Could you check a few things on this model? Use its own coordinates, in mm. A direction names the side the tool comes from. Give positions to 0.01 mm unless a question says otherwise; leave off trailing zeros. Loops run counter-clockwise (first coordinate to the right, second up) from the corner with the lowest first, then second, coordinate; pieces in that order, holes last. Notation, with made-up numbers: (12, 40) - (59, 40) arc R38 cw to (59, 78) - close; hole circle Ø11 at (20, 2.25). An arc over 180 degrees is marked (long way). Write each question's results on one line, items separated by ' | '. Start each with the question number.
1) If I drill on probe 1 along Z at (x, y) = (-30.5, 0.5); probe 2 along X at (y, z) = (-2.5, 0.7) (3 decimals); probe 3 along X at (y, z) = (-4.25, 2.55), over which ranges is the centre line in solid material (lowest first)? Write a range as [from, to].
2) If we mould it in two halves opening along X, with no side actions, what happens to faces 1 (the face through (-47, 0, 1)), 2 (the face through (-1.7, -3.2, 1)), 3 (the face through (-38, -5, 2))? For each: +X half, -X half, draft (parallel to the pull), parting line (faces both ways), or undercut.
3) I want a section at B-B, the plane y = 0.5. Write out the boundary of the cut face in (x, z), and give its area (3 significant figures).
4) I want a section at C-C, the plane y = -1.5. Write out the boundary of the cut face in (x, z).
5) I want a section at A-A, the plane z = 1.35. Count the separate pieces of the cut face and the enclosed holes in it, and give its area (3 significant figures).
6) I want a section at D-D, the plane y = 2.5. Write out the boundary of the cut face in (x, z) (3 decimals), and give its area (3 significant figures).
7) On a 3-axis mill with a long thin cutter (end or side, diameter ignored), from which of +Z, -Z, +X, -X, +Y, -Y can I reach the whole of each face in a straight line? I mean faces 4 (the face through (-3, -5, 1)), 5 (the face through (-42, -4, 3)), 6 (the face through (-35, -4, 3)). Say none if no direction works.
8) I'm going to push a flat-ended pin straight in: pin 1 (2.5 mm diameter, centred on x = -9.625, y = 0, fed in from +Z). Where does the tip first touch, or does it pass through?
from build123d import *

# Parameters (mm, degrees)
BOSS_EXTRUDE1_DEPTH = 2
SKETCH3_R           = 3.625
SKETCH3_R_2         = 1
CUT_EXTRUDE1_DEPTH  = 2
SKETCH4_W           = 7
SKETCH4_H           = 4
BOSS_EXTRUDE2_DEPTH = 3
SKETCH7_R           = 2
CUT_EXTRUDE2_DEPTH  = 7


with BuildPart() as part:
    # Sketch1 → Boss-Extrude1 (new body)
    with BuildSketch(Plane.XY):
        with BuildLine():
            Line((-42, 5), (0, 5))
            ThreePointArc((0, 5), (5, 0), (0, -5))
            Line((0, -5), (-42, -5))
            ThreePointArc((-42, -5), (-47, 0), (-42, 5))
        make_face()
    extrude(amount=BOSS_EXTRUDE1_DEPTH)

    # Sketch3 → Cut-Extrude1 (cut)
    with BuildSketch(Plane(origin=(0, 0, 0), x_dir=(-1, 0, 0), z_dir=(0, 0, -1))):
        with BuildLine():
            Line((6.625, -5), (35, -5))
            ThreePointArc((35, -5), (20.8125, 0), (6.625, -5))
        make_face()
        Circle(SKETCH3_R)
        with Locations((6.625, 0)):
            Circle(SKETCH3_R_2)
        with Locations((9.625, 0)):
            Circle(SKETCH3_R_2)
        with Locations((12.625, 0)):
            Circle(SKETCH3_R_2)
    extrude(amount=-CUT_EXTRUDE1_DEPTH, mode=Mode.SUBTRACT)

    # Sketch4 → Boss-Extrude2 (add)
    with BuildSketch(Plane.XZ.offset(5)):
        with Locations((-38.5, 2)):
            Rectangle(SKETCH4_W, SKETCH4_H)
    extrude(amount=-BOSS_EXTRUDE2_DEPTH)

    # Sketch7 → Cut-Extrude2 (cut)
    with BuildSketch(Plane.ZY.offset(42)):
        with Locations((4, -2)):
            Circle(SKETCH7_R)
    extrude(amount=-CUT_EXTRUDE2_DEPTH, mode=Mode.SUBTRACT)


solid = part.part
Answers:
1) probe 1: z = [0, 2] | probe 2: x = [-46.33, -31.151], [-10.474, -2.625], [2.625, 4.33] | probe 3: x = [-42, -35]
2) face 1: -X half | face 2: undercut | face 3: draft
3) outline: (-46.97, 0) - (-13.49, 0) - (-13.49, 2) - (-46.97, 2) - close; (-11.76, 0) - (-10.49, 0) - (-10.49, 2) - (-11.76, 2) - close; (-8.76, 0) - (-7.49, 0) - (-7.49, 2) - (-8.76, 2) - close; (-5.76, 0) - (-3.59, 0) - (-3.59, 2) - (-5.76, 2) - close; (3.59, 0) - (4.97, 0) - (4.97, 2) - (3.59, 2) - close | area: 79.1 mm2
4) outline: (-46.77, 0) - (-28.91, 0) - (-28.91, 2) - (-46.77, 2) - close; (-12.71, 0) - (-3.3, 0) - (-3.3, 2) - (-12.71, 2) - close; (3.3, 0) - (4.77, 0) - (4.77, 2) - (3.3, 2) - close
5) separate pieces: 1 | enclosed holes: 4 | area: 351 mm2
6) outline: (-46.33, 0) - (-2.625, 0) - (-2.625, 2) - (-46.33, 2) - close; (2.625, 0) - (4.33, 0) - (4.33, 2) - (2.625, 2) - close | area: 90.8 mm2
7) face 4: +Z, -Z, +X, -X, -Y | face 5: +Z, -X, +Y, -Y | face 6: +Z, +X, +Y, -Y
8) pin 1: stops at z = 2
